```python
from build123d import *

# Parameters (mm, degrees)
SKETCH_1_W          = 250
SKETCH_1_H          = 125
EXTRUDE_1_DEPTH     = 15
SHELL_1_T           = 1.2
CUT_EXTRUDE_1_REACH = 142.557
SKETCH_3_W          = 230
SKETCH_3_H          = 105


with BuildPart() as part:
    # 草图1 → 凸台-拉伸1 (new body)
    with BuildSketch(Plane.XY):
        Rectangle(SKETCH_1_W, SKETCH_1_H)
    extrude(amount=EXTRUDE_1_DEPTH)

    # 抽壳1 (no face opened: a closed hollow body)
    add(offset(amount=-SHELL_1_T, mode=Mode.PRIVATE), mode=Mode.SUBTRACT)

    # 草图3 → 切除-拉伸1 (cut, up to next)
    with BuildSketch(Plane.XY.offset(15), mode=Mode.PRIVATE) as cut_extrude_1_sk1:
        Rectangle(SKETCH_3_W, SKETCH_3_H)
    cut_extrude_1_tool1 = extrude(cut_extrude_1_sk1.sketch, amount=-CUT_EXTRUDE_1_REACH, mode=Mode.PRIVATE) & part.part
    add(cut_extrude_1_tool1.solids().sort_by_distance((0, 0, 15))[0], mode=Mode.SUBTRACT)


solid = part.part
```
Geometry check sheet. Reference: the model listing, model coordinates, mm. A direction names the side the tool comes from. Coordinates: 2 decimals unless noted, no trailing zeros. Write each loop counter-clockwise with the first axis right and the second up, starting at its lowest first coordinate (ties: lowest second). Pieces come first, ordered by that corner, then holes. Notation, with made-up numbers: M 41,28 L 75,28 A26 cw 75,62 Z; hole C 69,87 d2. An arc over 180 degrees is marked long. Answer as a JSON object with one key per item and string values.
1. Section check B-B, the plane y = -15.5. Enter the section's corners in (x, z), plus the area to 3 significant figures.
Answers below:
{"outline": "M -125,0 L 125,0 L 125,15 L 115,15 L 115,13.8 L 123.8,13.8 L 123.8,1.2 L -123.8,1.2 L -123.8,13.8 L -115,13.8 L -115,15 L -125,15 Z", "area": "354 mm²"}
2. Section check A-A, the plane z = 4.5. Enter the section's corners in (x, y).
Answers below:
{"outline": "M -125,-62.5 L 125,-62.5 L 125,62.5 L -125,62.5 Z; hole M -123.8,-61.3 L 123.8,-61.3 L 123.8,61.3 L -123.8,61.3 Z"}
3. Scan lines: L1, parallel to X at y = -38, z = 3.25; L2, parallel to Y at x = 64.5, z = 6.25; L3, parallel to X at y = -4.5, z = 14.5. Record each from-to range of solid material in increasing order.
Answers below:
{"L1": "x = -125 to -123.8, 123.8 to 125", "L2": "y = -62.5 to -61.3, 61.3 to 62.5", "L3": "x = -125 to -115, 115 to 125"}
4. Tool access check on faces 5 (the flat face through (-125, -1, 7)), 6 (the flat face through (-2, -61.3, 7)). Record the directions out of +Z, -Z, +X, -X, +Y, -Y that give a thin tool (end or side, any length) a straight path to the whole face; none if there is none.
Answers below:
{"face 5": "+Z, -Z, -X, +Y, -Y", "face 6": "none"}
5. Section check C-C, the plane x = -64.5. Enter the section's corners in (y, z).
Answers below:
{"outline": "M -62.5,0 L 62.5,0 L 62.5,15 L 52.5,15 L 52.5,13.8 L 61.3,13.8 L 61.3,1.2 L -61.3,1.2 L -61.3,13.8 L -52.5,13.8 L -52.5,15 L -62.5,15 Z"}
6. Go/stop test with flat-tipped pins: pin 1 Ø3 at (x, y) = (-18.5, 16.5) entering from +Z; pin 2 Ø1.5 at (x, y) = (3, 10) entering from -Z. Record where each tip stops, or that it passes through.
Answers below:
{"pin 1": "stops at z = 1.2", "pin 2": "stops at z = 0"}
7. Draft check along X on faces 1 (the flat face through (-2, 61.3, 7)), 2 (the flat face through (125, -1, 7)), 3 (the flat face through (123.8, -1, 7)), 4 (the flat face through (-10, -55, 15)). Enter one of: released by +X, released by -X, zero draft, split by the parting line, or undercut.
Answers below:
{"face 1": "undercut", "face 2": "released by +X", "face 3": "undercut", "face 4": "zero draft"}
